Could you check a few things on this model? Use its own coordinates, in mm. A direction names the side the tool comes from. Give positions to 0.01 mm unless a question says otherwise; leave off trailing zeros. Order: outer loops, then holes, each group sorted by start corner. A loop starts at its lowest first (then second) coordinate and runs counter-clockwise, first axis right, second up. Notation, with made-up numbers: (-20, 78.25) - (-15, 78.25) arc R32 ccw to (-15, 110.25) - close; hole circle Ø1 at (7.5, 25.25). An arc over 180 degrees is marked (long way). Put each result on its own line as item: value.
from build123d import *

# Parameters (mm, degrees)
BOSS_EXTRUDE2_DEPTH = 135.89
RIB18_REACH         = 308.18
SKETCH4_WALL_W      = 743.085279388
SKETCH4_WALL_H      = 5.08
RIB27_REACH         = 197.826
SKETCH6_WALL_W      = 574.331256006
SKETCH6_WALL_H      = 5.08


with BuildPart() as part:
    # Sketch1 → Boss-Extrude2 (new, symmetric)
    with BuildSketch(Plane(origin=(0, 0, 0), x_dir=(1, 0, 0), z_dir=(0, 1, 0))):
        Polygon((-11.562777715, 77.955501368), (0, 77.955501368), (0, -59.305859892), (117.492741296, -59.305859892), (117.492741296, -69.749659119), (-11.562777715, -69.749659119), (-11.562777715, -59.305859892), align=None)
    extrude(amount=BOSS_EXTRUDE2_DEPTH, both=True)

    # Sketch4 wall → Rib18 (add, up to next)
    with BuildSketch(Plane(origin=(29.373185324, 135.89, 2.036221127), x_dir=(0.456367573522, 0, 0.889791345113), z_dir=(0.889791345113, 0, -0.456367573522)), mode=Mode.PRIVATE) as rib18_sk1:
        with Locations((0, 2.54)):
            Rectangle(SKETCH4_WALL_W, SKETCH4_WALL_H)
    rib18_tool1 = extrude(rib18_sk1.sketch, amount=-RIB18_REACH, mode=Mode.PRIVATE) - part.part
    add(rib18_tool1.solids().sort_by_distance((29.373185324, 135.89, 2.036221127))[0])

    # Sketch6 wall → Rib27 (add, up to next)
    with BuildSketch(Plane(origin=(58.746370648, 0, -9.324820738), x_dir=(0.650281202153, 0, 0.759693594896), z_dir=(0.759693594896, 0, -0.650281202153)), mode=Mode.PRIVATE) as rib27_sk1:
        Rectangle(SKETCH6_WALL_W, SKETCH6_WALL_H)
    rib27_tool1 = extrude(rib27_sk1.sketch, amount=-RIB27_REACH, mode=Mode.PRIVATE) - part.part
    add(rib27_tool1.solids().sort_by_distance((58.746370648, 0, -9.324820738))[0])


solid = part.part
1) If I drill on line 1 (Y direction, x = 6, z = 8); line 2 (Y direction, x = 51, z = 40.5); line 3 (Z direction, x = 112.5, y = 74), over which ranges is the centre line in solid material (lowest first)? Write a range as [from, to].
Filled in:
line 1: y = [-2.54, 2.54], [130.81, 135.89]
line 2: y = [-2.54, 2.54]
line 3: z = [59.31, 69.75]
2) Suppose I cut it at A-A, the plane y = -17. List the corners of the cut face in (x, z) for me, and give its area (3 significant figures).
Filled in:
outline: (-11.56, -77.96) - (0, -77.96) - (0, 59.31) - (117.49, 59.31) - (117.49, 69.75) - (-11.56, 69.75) - close
area: 2,930 mm^2
3) Which directions (+Z, -Z, +X, -X, +Y, -Y) give clear straight access to the entire face, cutting with the end or side of a thin tool? Please do faces 4 (the flat face through (0, -68, -10)), 5 (the flat face through (40, 2.54, 5)), 6 (the flat face through (28.96, 133.31, 1.23)), 7 (the flat face through (-6, 2, -77.956)).
Filled in:
face 4: -Z, +X, -Y
face 5: -Z, +X
face 6: -Z, +X, +Y
face 7: -Z, +X, -X, +Y, -Y
4) Suppose I cut it at D-D, the plane x = 79.5. List the corners of the cut face in (y, z) for me.
Filled in:
outline: (-135.89, 59.31) - (-2.54, 59.31) - (-2.54, 14.92) - (2.54, 14.92) - (2.54, 59.31) - (135.89, 59.31) - (135.89, 69.75) - (-135.89, 69.75) - close
5) Suppose I cut it at B-B, the plane z = -52. List the corners of the cut face in (x, y) for me, and give its area (3 significant figures).
Filled in:
outline: (-11.56, -135.89) - (0, -135.89) - (0, -2.54) - (22.22, -2.54) - (22.22, 2.54) - (0, 2.54) - (0, 130.81) - (1.66, 130.81) - (1.66, 135.89) - (-11.56, 135.89) - close
area: 3,260 mm^2
6) We'd pull the mould along Y, two halves only. Please class faces 1 (the flat face through (24, 135.89, 26)), 2 (the flat face through (58, 70, 59.306)), 3 (the flat face through (-4, -135.89, 28)): pulls with the +Y half, pulls with the -Y half, needs draft (parallel to the pull), parting line crosses it, or undercut.
Filled in:
face 1: pulls with the +Y half
face 2: undercut
face 3: pulls with the -Y half
7) Suppose I cut it at C-C, the plane x = 47. List the corners of the cut face in (y, z) for me, and give its area (3 significant figures).
Filled in:
outline: (-135.89, 59.31) - (-2.54, 59.31) - (-2.54, -23.05) - (2.54, -23.05) - (2.54, 59.31) - (130.81, 59.31) - (130.81, 36.4) - (135.89, 36.4) - (135.89, 69.75) - (-135.89, 69.75) - close
area: 3,370 mm^2
8) I'm going to push flat-ended pins straight in: pin 1 (10 mm diameter, centred on y = 90, z = -50, fed in from +X); pin 2 (8 mm diameter, centred on x = 94, y = -45, fed in from -Z); pin 3 (2 mm diameter, centred on x = 16, z = -62, fed in from -Y). Where does each tip first touch, or does it pass through?
Filled in:
pin 1: stops at x = 0
pin 2: stops at z = 59.31
pin 3: passes through
